Source: CAD feature listing. Evaluate the final solid. Frame: model axes, mm. A direction names the side the tool comes from. Coordinates: 2 decimals unless noted, no trailing zeros. Write each loop counter-clockwise with the first axis right and the second up, starting at its lowest first coordinate (ties: lowest second). Pieces come first, ordered by that corner, then holes. Notation, with made-up numbers: M 6,70.25 L 43,70.25 A23 ccw 43,93.25 Z; hole C 78,69 d2. An arc over 180 degrees is marked long. Answer as CSV lines item,"result". Start each with the question number.
1. Contact query for a flat-ended pin moving along its axis: pin 1 Ø3 at (x, z) = (-198.5, -7.5) entering from +Y. Output: stop coordinate, or through.
2. Mould query, pull axis Z, two halves, no side actions, for faces 6 (the face through (-380, 20, 1)), 7 (the face through (-5, 20, -49.1)), 8 (the face through (-38, 20, -19.1)). Classes: pulls with the +Z half, pulls with the -Z half, needs draft (parallel to the pull), parting line crosses it, or undercut.
3. Reachability of faces 1 (the face through (-5, 20, 49.1)), 2 (the face through (-5, 0, 1)), 3 (the face through (-342.605, 38.167, 2.343)), 4 (the face through (350, 21, 0)), 5 (the face through (-38, 20, 19.1)) from +Z, -Z, +X, -X, +Y, -Y: full face, straight path, thin tool, end or side. Return the list, or none.
4. Line query: probe 1 along Y at (x, z) = (-344.5, 0); probe 2 along Z at (x, y) = (146.5, 29.5); probe 3 along X at (y, z) = (22.5, 15.5). Output: solid intervals per line, ascending. Write a range as [from, to].
5. Section C-C on x = 251.5. Return the cut outline in (y, z), plus the area to 3 significant figures.
6. Section B-B on y = 20.32. Return the cut outline in (x, z), plus the area to 3 significant figures.
7. Section A-A on z = 0. Return the cut outline in (x, y).
```python
from build123d import *

# Parameters (mm, degrees)
SKETCH1_W           = 760
SKETCH1_H           = 98.2
SKETCH1_W_2         = 700
SKETCH1_H_2         = 38.2
BOSS_EXTRUDE3_DEPTH = 40.64
SKETCH2_W           = 700
SKETCH2_H           = 38.2
BOSS_EXTRUDE4_DEPTH = 0.254
SKETCH3_W           = 67.5
SKETCH3_H           = 43.5
CUT_EXTRUDE1_DEPTH  = 40.386
CUT_EXTRUDE5_REACH  = 387.308
SKETCH5_W           = 67.5
SKETCH5_H           = 43.5
SKETCH6_R           = 18
SKETCH6_R_2         = 12.8397
BOSS_EXTRUDE5_DEPTH = 15


with BuildPart() as part:
    # Sketch1 → Boss-Extrude3 (new body)
    with BuildSketch(Plane(origin=(0, 0, 0), x_dir=(1, 0, 0), z_dir=(0, 1, 0))):
        Rectangle(SKETCH1_W, SKETCH1_H)
        Rectangle(SKETCH1_W_2, SKETCH1_H_2, mode=Mode.SUBTRACT)
    extrude(amount=BOSS_EXTRUDE3_DEPTH)

    # Sketch2 → Boss-Extrude4 (add)
    with BuildSketch(Plane.XZ):
        Rectangle(SKETCH2_W, SKETCH2_H)
    extrude(amount=-BOSS_EXTRUDE4_DEPTH)

    # Sketch3 → Cut-Extrude1 (cut)
    with BuildSketch(Plane(origin=(0, 40.64, 0), x_dir=(1, 0, 0), z_dir=(0, 1, 0))):
        with Locations((316.25, 0)):
            Rectangle(SKETCH3_W, SKETCH3_H)
    extrude(amount=-CUT_EXTRUDE1_DEPTH, mode=Mode.SUBTRACT)

    # Sketch5 → Cut-Extrude5 (cut, up to next)
    with BuildSketch(Plane(origin=(0, 40.64, 0), x_dir=(1, 0, 0), z_dir=(0, 1, 0)), mode=Mode.PRIVATE) as cut_extrude5_sk1:
        with Locations((316.25, 0)):
            Rectangle(SKETCH5_W, SKETCH5_H)
    cut_extrude5_tool1 = extrude(cut_extrude5_sk1.sketch, amount=-CUT_EXTRUDE5_REACH, mode=Mode.PRIVATE) & part.part
    add(cut_extrude5_tool1.solids().sort_by_distance((316.25, 40.64, 0))[0], mode=Mode.SUBTRACT)

    # Sketch6 → Boss-Extrude5 (add)
    with BuildSketch(Plane(origin=(-350, 0, 0), x_dir=(0, 0, -1), z_dir=(1, 0, 0))):
        with Locations((0, 20.32)):
            Circle(SKETCH6_R)
        with Locations((0, 20.32)):
            Circle(SKETCH6_R_2, mode=Mode.SUBTRACT)
    extrude(amount=BOSS_EXTRUDE5_DEPTH)


solid = part.part
```
Values:
1,pin 1,"y = 0.25"
2,face 6,"needs draft"
2,face 7,"pulls with the -Z half"
2,face 8,"undercut"
3,face 1,"+Z, +X, -X, +Y, -Y"
3,face 2,"+Z, -Z, +X, -X, -Y"
3,face 3,"none"
3,face 4,"+Y, -Y"
3,face 5,"+Y"
4,probe 1,"[0, 0.25], [2.32, 7.48], [33.16, 38.32]"
4,probe 2,"[-49.1, -19.1], [19.1, 49.1]"
4,probe 3,"[-380, -335], [350, 380]"
5,outline,"M 0,-49.1 L 40.64,-49.1 L 40.64,-19.1 L 0.25,-19.1 L 0.25,19.1 L 40.64,19.1 L 40.64,49.1 L 0,49.1 Z"
5,area,"2,450 mm²"
6,outline,"M -380,-49.1 L 380,-49.1 L 380,49.1 L -380,49.1 Z; hole M -350,-19.1 L 282.5,-19.1 L 282.5,-21.75 L 350,-21.75 L 350,21.75 L 282.5,21.75 L 282.5,19.1 L -350,19.1 L -350,18 L -335,18 L -335,12.84 L -350,12.84 L -350,-12.84 L -335,-12.84 L -335,-18 L -350,-18 Z"
6,area,"47,700 mm²"
7,outline,"M -380,0 L 282.5,0 L 282.5,0.25 L -350,0.25 L -350,2.32 L -335,2.32 L -335,7.48 L -350,7.48 L -350,33.16 L -335,33.16 L -335,38.32 L -350,38.32 L -350,40.64 L -380,40.64 Z; M 350,0 L 380,0 L 380,40.64 L 350,40.64 Z"
